```python
from build123d import *

# Parameters (mm, degrees)
F0_R           = 25
F0_R_2         = 13.75
F1_DEPTH       = 7
F2_DEPTH       = 78
F3_D           = 4.5
F3_CBORE_D     = 8.25
F3_CBORE_DEPTH = 4.5
F4_R           = 1


with BuildPart() as f1:
    # F0 (on Top) → F1 (new body)
    with BuildSketch(Plane.XY):
        Circle(F0_R)
        Circle(F0_R_2, mode=Mode.SUBTRACT)
    extrude(amount=F1_DEPTH)

    # F0 (on Top) → F2 (join)
    with BuildSketch(Plane.XY):
        Circle(F0_R_2)
    extrude(amount=F2_DEPTH)

    # F3 (through all)
    with Locations(Plane(origin=(0, 0, 0), x_dir=(1, 0, 0), z_dir=(0, 0, -1))):
        with Locations((3.0853754045, 17.2258659757), (13.3753498349, -11.2849464684), (-16.4607252394, -5.9409195073)):
            CounterBoreHole(F3_D / 2, F3_CBORE_D / 2, F3_CBORE_DEPTH)

    # F4
    f4_edges = [f1.edges().sort_by_distance(p)[0] for p in [
        (-25, 0, 7),
    ]]
    fillet(f4_edges, radius=F4_R)


solid = f1.part
```
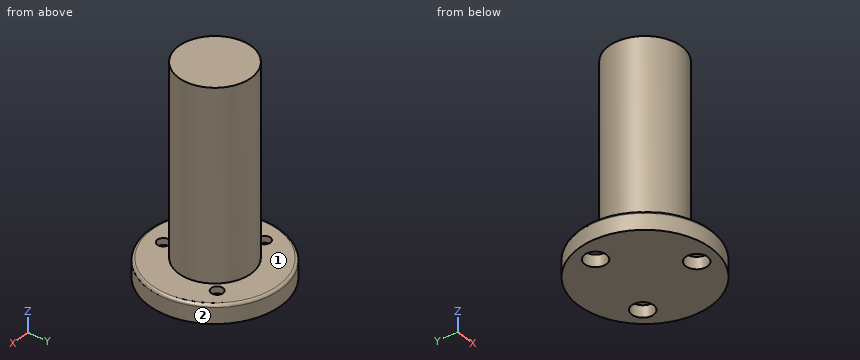
The listing builds one solid part. Answer for the finished solid, in the listing's coordinates (mm). Face numbers are marked on the shaded views. A direction names the side the tool comes from. Coordinates: 2 decimals unless noted, no trailing zeros. Loops run counter-clockwise (first coordinate to the right, second up) from the corner with the lowest first, then second, coordinate; pieces in that order, holes last. Notation, with made-up numbers: (12.5, -22) - (23.5, -22) arc R21 cw to (23.5, 13) - close; hole circle Ø6 at (64.5, -31.5). An arc over 180 degrees is marked (long way). Use a Markdown table: item, result. Add a question column.
1) Given pin 1 (5 mm diameter, centred on x = 13.38, y = 11.28, fed in from -Z); pin 2 (8 mm diameter, centred on x = -1.5, z = 62.5, fed in from +Y); pin 3 (6.5 mm diameter, centred on x = -16.46, y = 5.94, fed in from +Z), each flat-ended and moving along its own axis, determine where each tip first touches the part or whether it passes through.
2) The part is cut by section B-B, the plane z = 49. Give the vertices of the cut face in (x, y), and give its area (3 significant figures).
3) For the marked faces 1 and 2, determine the directions among +Z, -Z, +X, -X, +Y, -Y from which every point of the face is accessible in a straight line to the end or side of a thin tool.
4) The part is cut by section A-A, the plane y = 0. Give the vertices of the cut face in (x, z), and give its area (3 significant figures).
5) Find the intervals of material crossed by line 1 (Z direction, x = 16, y = -4); line 2 (Y direction, x = -4.5, z = 24.5); line 3 (X direction, y = 8.5, z = 73), in increasing order.
Here are the results:
| question | item | result |
|---|---|---|
| 1 | pin 1 | stops at z = 4.5 |
| 1 | pin 2 | stops at y = 13.75 |
| 1 | pin 3 | stops at z = 7 |
| 2 | outline | circle Ø27.5 at (0, 0) |
| 2 | area | 594 mm^2 |
| 3 | face 1 | +Z |
| 3 | face 2 | +Z, -Z |
| 4 | outline | (-25, 0) - (25, 0) - (25, 6) arc R1 ccw to (24, 7) - (13.75, 7) - (13.75, 78) - (-13.75, 78) - (-13.75, 7) - (-24, 7) arc R1 ccw to (-25, 6) - close |
| 4 | area | 2,300 mm^2 |
| 5 | line 1 | z = 0 to 7 |
| 5 | line 2 | y = -12.99 to 12.99 |
| 5 | line 3 | x = -10.81 to 10.81 |
